from build123d import *

# Parameters (mm, degrees)
SKETCH1_R           = 2.0193
SKETCH1_R_2         = 14.195
BOSS_EXTRUDE1_DEPTH = 2.413
BOSS_EXTRUDE2_DEPTH = 29.21
BOSS_EXTRUDE9_DEPTH = 16.51
FILLET1_R           = 1.27


with BuildPart() as part:
    # Sketch1 → Boss-Extrude1 (new body)
    with BuildSketch(Plane.XY):
        with BuildLine():
            Line((-21, 14.827700733), (-21, -20))
            Line((-21, -20), (-20, -21))
            Line((-20, -21), (26.136694206, -21))
            Line((26.136694206, -21), (26.9748, -19.911980036))
            Line((26.9748, -19.911980036), (26.9748, 0))
            Line((26.9748, 0), (26.637921908, 20.360449416))
            ThreePointArc((26.637921908, 20.360449416), (-0.633988092, 33.522005356), (-27.388735161, 19.338665163))
            Line((-27.388735161, 19.338665163), (-21, 14.827700733))
        make_face()
        with Locations((-17.960512242, 17.960512242)):
            Circle(SKETCH1_R, mode=Mode.SUBTRACT)
        with Locations((17.960512242, -17.960512242)):
            Circle(SKETCH1_R, mode=Mode.SUBTRACT)
        Circle(SKETCH1_R_2, mode=Mode.SUBTRACT)
    extrude(amount=BOSS_EXTRUDE1_DEPTH)

    # Sketch2 → Boss-Extrude2 (add)
    with BuildSketch(Plane.XY.offset(2.413)):
        with BuildLine():
            Line((-26.362552713, 18.590168866), (-27.400448489, 19.322065278))
            ThreePointArc((-27.400448489, 19.322065278), (-0.644144472, 33.521811734), (26.637921908, 20.360449416))
            Line((26.637921908, 20.360449416), (25.628909714, 19.589220272))
            ThreePointArc((25.628909714, 19.589220272), (-0.619745061, 32.252046138), (-26.362552713, 18.590168866))
        make_face()
    extrude(amount=BOSS_EXTRUDE2_DEPTH)

    # Sketch3 → Boss-Extrude9 (add)
    with BuildSketch(Plane.XY.offset(2.413)):
        with BuildLine():
            Line((-23.55281498, 18.123360163), (-25.598477532, 19.628971243))
            ThreePointArc((-25.598477532, 19.628971243), (-25.979914408, 19.121260716), (-26.351283072, 18.606139967))
            Line((-26.351283072, 18.606139967), (-24.25635866, 17.12695367))
            Line((-24.25635866, 17.12695367), (-23.55281498, 18.123360163))
        make_face()
        with BuildLine():
            Line((-1.244999497, 25.907990312), (-1.244999497, 32.23396563))
            ThreePointArc((-1.244999497, 32.23396563), (-0.610117761, 32.252229695), (0.025000503, 32.257990312))
            Line((0.025000503, 32.257990312), (0.025000503, 25.907990312))
            Line((0.025000503, 25.907990312), (-1.244999497, 25.907990312))
        make_face()
        Polygon((25.628909714, 19.589220272), (25.628909714, 11.969220272), (26.776760752, 11.969220272), (26.637921908, 20.360449416), align=None)
    extrude(amount=BOSS_EXTRUDE9_DEPTH)

    # Fillet1
    fillet1_edges = [part.edges().sort_by_distance(p)[0] for p in [
        (-24.194367581, 17.083182948, 0),
        (-26.881500601, 18.956117072, 31.623),
        (26.133415811, 19.974834844, 31.623),
    ]]
    fillet(fillet1_edges, radius=FILLET1_R)


solid = part.part
The listing builds one solid part. Answer for the finished solid, in the listing's coordinates (mm). A direction names the side the tool comes from. Coordinates: 2 decimals unless noted, no trailing zeros. Order: outer loops, then holes, each group sorted by start corner. A loop starts at its lowest first (then second) coordinate and runs counter-clockwise, first axis right, second up.
Q1. A cutting plane is placed at A-A, the plane y = 10. Write down the section's boundary in (x, z), and give its area (3 significant figures).
Q2. A cutting plane is placed at B-B, the plane z = 7. Write down the section's boundary in (x, y) (3 decimals), and give its area (3 significant figures).
Q3. Which of the six approach directions +Z, -Z, +X, -X, +Y, -Y give full straight-line access (tool end or side, diameter ignored) to faces 1 (the face through (-3.077, -13.857, 1.19)), 2 (the face through (-1, 25.908, 11)), 3 (the face through (-24.561, 18.866, 10.552))?
Q4. A cutting plane is placed at C-C, the plane x = -7. Write down the section's boundary in (y, z), and give its area (3 significant figures).
Q5. Given P1, Ø0.9, axis at x = 26, y = 15.5, coming from the +Z side; P2, Ø2.5, axis at y = 17, z = 7.5, coming from the -X side; P3, Ø1.3, axis at x = 26.5, z = 9, coming from the -Y side; P4, Ø10, axis at x = -16, y = 16.5, coming from the -Z side, each flat-ended and moving along its own axis, determine where each tip first touches the part or whether it passes through.
Q6. A cutting plane is placed at D-D, the plane y = -10.5. Write down the section's boundary in (x, z), and give its area (3 significant figures).
Q7. For a pull along X with two mould halves and no side action, classify faces 4 (the face through (26.975, -10, 1)), 5 (the face through (12, 13, 0)), 6 (the face through (25.629, 16, 11)) as pulls with the +X half, pulls with the -X half, needs draft (parallel to the pull), parting line crosses it, or undercut.
Q8. Consider line 1 (Y direction, x = 0, z = 1.1) (3 decimals); line 2 (Z direction, x = 17, y = 19); line 3 (Y direction, x = -11, z = 2). Determine where each line is inside the solid, lowest interval first.
Answers follow:
1. outline: (-21, 0) - (-10.07, 0) - (-10.07, 2.41) - (-21, 2.41) - close; (10.07, 0) - (26.81, 0) - (26.81, 2.41) - (10.07, 2.41) - close
1. area: 66.7 mm2
2. outline: (-27.4, 19.322) - (-26.363, 18.59) arc R32.258 cw to (-26.351, 18.606) - (-24.256, 17.127) - (-23.553, 18.123) - (-25.598, 19.629) arc R32.258 cw to (-1.245, 32.234) - (-1.245, 25.908) - (0.025, 25.908) - (0.025, 32.258) arc R32.258 cw to (25.629, 19.589) - (25.629, 11.969) - (26.777, 11.969) - (26.638, 20.36) arc R33.528 ccw to start
2. area: 98.2 mm2
3. face 1: +Z, -Z
3. face 2: +Z, -Y
3. face 3: +Z
4. outline: (-21, 0) - (-12.35, 0) - (-12.35, 2.41) - (-21, 2.41) - close; (12.35, 0) - (32.79, 0) - (32.79, 31.62) - (31.49, 31.62) - (31.49, 2.41) - (12.35, 2.41) - close
4. area: 108 mm2
5. P1: stops at z = 18.92
5. P2: stops at x = -25.85
5. P3: stops at y = 11.97
5. P4: stops at z = 0
6. outline: (-21, 0) - (-9.55, 0) - (-9.55, 2.41) - (-21, 2.41) - close; (9.55, 0) - (26.97, 0) - (26.97, 2.41) - (9.55, 2.41) - close
6. area: 69.7 mm2
7. face 4: pulls with the +X half
7. face 5: needs draft
7. face 6: undercut
8. line 1: y = -21 to -14.195, 14.195 to 33.528
8. line 2: z = 0 to 2.41
8. line 3: y = -21 to -8.97, 8.97 to 31.67
